Input: part model. Units: mm. Frame: model coordinates. Face numbers are marked on the shaded views. A direction names the side the tool comes from. Round coordinates to 2 decimals unless told otherwise and drop trailing zeros. Order: outer loops, then holes, each group sorted by start corner. A loop starts at its lowest first (then second) coordinate and runs counter-clockwise, first axis right, second up.
Item 1: Line query: L1, parallel to X at y = 0, z = 4.8 (3 decimals); L2, parallel to X at y = 0, z = 6.75; L3, parallel to Z at x = 15, y = 11. Output: solid intervals per line, ascending.
Item 2: Cut plane D-D on y = -17. Output: boundary loops of the cut face in (x, z), then the cut area to 3 significant figures.
Item 3: Cut plane C-C on z = 4. Give the number of separate pieces and of enclosed holes in the cut face, then the cut area to 3 significant figures.
Item 4: Reachability of the marked faces 4, 5, 6 and 7 from +Z, -Z, +X, -X, +Y, -Y: full face, straight path, thin tool, end or side. Return the list, or none.
Item 5: Cut plane B-B on y = 0. Output: boundary loops of the cut face in (x, z) (3 decimals).
Item 6: Cut plane A-A on x = 0. Output: boundary loops of the cut face in (y, z) (3 decimals).
Item 7: First-contact query: pin 1 (1 mm diameter, centred on x = -3, y = 9.5, fed in from +Z); pin 2 (10 mm diameter, centred on x = 2.5, z = 10.5, fed in from -Y); pin 3 (8 mm diameter, centred on y = 7.5, z = 18, fed in from +X). Flat tips, straight axial feed; report the tip coordinate or a pass-through.
Item 8: Mould query, pull axis Y, two halves, no side actions, for the marked faces 1, 2 and 3. Classes: released by +Y, released by -Y, zero draft, split by the parting line, or undercut.
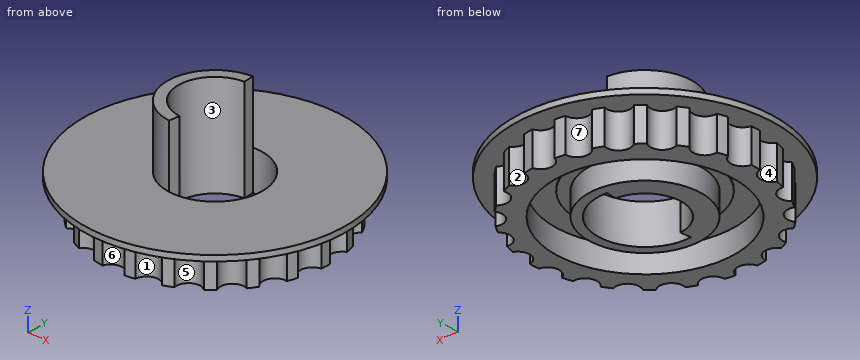
```python
from build123d import *

# Parameters (mm, degrees)
SKETCH006_R        = 20.3333820507
PAD006_DEPTH       = 6
SKETCH007_R        = 2.1
POCKET_DEPTH       = 121.6482464863
POLARPATTERN_COUNT = 22
SKETCH013_R        = 23.2333820507
PAD007_DEPTH       = 1
SKETCH008_R        = 16
SKETCH008_R_2      = 10.075
POCKET001_DEPTH    = 4.2
SKETCH014_R        = 12
PAD008_DEPTH       = 0.2
SKETCH015_R        = 8.4
POCKET002_DEPTH    = 7.001
PAD009_DEPTH       = 18


with BuildPart() as part:
    # Sketch006 → Pad006 (new body)
    with BuildSketch(Plane.XY):
        Circle(SKETCH006_R)
    extrude(amount=PAD006_DEPTH)

    # Sketch007 (on Face3 of Pad006) → Pocket (cut, through all)
    with BuildSketch(Plane.XY.offset(6)):
        with Locations((0, 20.8333820507)):
            Circle(SKETCH007_R)
    pocket = extrude(amount=-POCKET_DEPTH, mode=Mode.SUBTRACT)

    # PolarPattern: Pocket ×22 about axis
    polarpattern_axis = Axis((0, 0, 6), (0, 0, 1))
    for i in range(1, POLARPATTERN_COUNT):
        add(pocket.rotate(polarpattern_axis, i * 360 / POLARPATTERN_COUNT), mode=Mode.SUBTRACT)

    # Sketch013 (on Face4 of PolarPattern) → Pad007 (join)
    with BuildSketch(Plane.XY.offset(6)):
        Circle(SKETCH013_R)
    extrude(amount=PAD007_DEPTH)

    # Sketch008 (on Face2 of PolarPattern) → Pocket001 (cut)
    with BuildSketch(Plane(origin=(0, 0, 0), x_dir=(1, 0, 0), z_dir=(0, 0, -1))):
        Circle(SKETCH008_R)
        Circle(SKETCH008_R_2, mode=Mode.SUBTRACT)
    extrude(amount=-POCKET001_DEPTH, mode=Mode.SUBTRACT)

    # Sketch014 (on Face51 of Pocket001) → Pad008 (join)
    with BuildSketch(Plane(origin=(0, 0, 4.2), x_dir=(1, 0, 0), z_dir=(0, 0, -1))):
        Circle(SKETCH014_R)
    extrude(amount=PAD008_DEPTH)

    # Sketch015 (on Face55 of Pad008) → Pocket002 (cut, through all)
    with BuildSketch(Plane(origin=(0, 0, 0), x_dir=(1, 0, 0), z_dir=(0, 0, -1))):
        Circle(SKETCH015_R)
    extrude(amount=-POCKET002_DEPTH, mode=Mode.SUBTRACT)

    # Sketch016 (on Face51 of Pocket002) → Pad009 (join)
    with BuildSketch(Plane(origin=(0, 0, 0), x_dir=(1, 0, 0), z_dir=(0, 0, -1))):
        with BuildLine():
            Line((-0.7321082391, -8.368035464), (-0.5665123279, -6.4752655376))
            ThreePointArc((-0.5665123279, 6.4752655376), (-6.5, 0), (-0.5665123279, -6.4752655376))
            Line((-0.7321082391, 8.368035464), (-0.5665123279, 6.4752655376))
            ThreePointArc((-0.7321082391, 8.368035464), (-8.4, 0), (-0.7321082391, -8.368035464))
        make_face()
    extrude(amount=-PAD009_DEPTH)


with BuildPart() as part_1:
    # Body001 placement: moved
    add(part.part.moved(Location((0, 0, 2.2))))


solid = part_1.part
```
From the geometry:
1. L1: x = -20.333 to -16, -10.075 to -6.5, 8.4 to 10.075, 16 to 20.333
1. L2: x = -20.33 to -6.5, 8.4 to 20.33
1. L3: z = 2.2 to 9.2
2. outline: (-15.84, 8.2) - (-9.23, 8.2) - (-9.23, 2.2) - (9.23, 2.2) - (9.23, 8.2) - (15.84, 8.2) - (15.84, 9.2) - (-15.84, 9.2) - close
2. area: 142 mm2
3. separate pieces: 2
3. enclosed holes: 2
3. area: 530 mm2
4. face 4: -Z, -X
4. face 5: -Z
4. face 6: -Z, -Y
4. face 7: -Z, +Y
5. outline: (-23.233, 8.2) - (-20.333, 8.2) - (-20.333, 2.2) - (-16, 2.2) - (-16, 6.4) - (-12, 6.4) - (-12, 6.2) - (-10.075, 6.2) - (-10.075, 2.2) - (-6.5, 2.2) - (-6.5, 20.2) - (-8.4, 20.2) - (-8.4, 9.2) - (-23.233, 9.2) - close; (8.4, 2.2) - (10.075, 2.2) - (10.075, 6.2) - (12, 6.2) - (12, 6.4) - (16, 6.4) - (16, 2.2) - (20.333, 2.2) - (20.333, 8.2) - (23.233, 8.2) - (23.233, 9.2) - (8.4, 9.2) - close
6. outline: (-23.233, 8.2) - (-18.733, 8.2) - (-18.733, 2.2) - (-16, 2.2) - (-16, 6.4) - (-12, 6.4) - (-12, 6.2) - (-10.075, 6.2) - (-10.075, 2.2) - (-8.4, 2.2) - (-8.4, 9.2) - (-23.233, 9.2) - close; (8.4, 2.2) - (10.075, 2.2) - (10.075, 6.2) - (12, 6.2) - (12, 6.4) - (16, 6.4) - (16, 2.2) - (18.733, 2.2) - (18.733, 8.2) - (23.233, 8.2) - (23.233, 9.2) - (8.4, 9.2) - close
7. pin 1: stops at z = 9.2
7. pin 2: stops at y = -23.23
7. pin 3: stops at x = -0.57
8. face 1: released by -Y
8. face 2: released by +Y
8. face 3: undercut
